The model under review builds one solid part; all positions refer to its coordinate system, in mm. A direction names the side the tool comes from. Coordinates: 2 decimals unless noted, no trailing zeros. Loops run counter-clockwise (first coordinate to the right, second up) from the corner with the lowest first, then second, coordinate; pieces in that order, holes last. Notation, with made-up numbers: (-25.75, 35.5) - (6.25, 35.5) arc R22 ccw to (6.25, 55.5) - close; hole circle Ø7 at (49.5, 52). An arc over 180 degrees is marked (long way). Use a Markdown table: item, result. Add a question column.
1) Add section B-B, the plane x = 205. Give the boundary of the cut face in (y, z), and give its area (3 significant figures).
2) Add section A-A, the plane z = -68. Give the boundary of the cut face in (x, y), and give its area (3 significant figures).
3) Add section C-C, the plane y = 62. Give the boundary of the cut face in (x, z).
4) Add section D-D, the plane z = -10. Give the boundary of the cut face in (x, y), and give its area (3 significant figures).
5) Clearance check with flat-ended pins moving along their axes: pin 1 (4 mm diameter, centred on x = 19.18, y = 96.25, fed in from -Z); pin 2 (1 mm diameter, centred on y = 67, z = 6, fed in from +X); pin 3 (4 mm diameter, centred on y = 31, z = -44.5, fed in from -X); pin 4 (10 mm diameter, centred on x = -85, z = -68, fed in from +Y). State where each tip first meets the part, or that it passes through.
6) To check wall thickness, follow L1, parallel to X at y = 39, z = -16; L2, parallel to Z at x = -150, y = 16; L3, parallel to Z at x = -205, y = 5. State the ranges of each line that lie inside material, in increasing order. Write a range as [from, to].
7) For faces 1 (the flat face through (-3, 62, -55)), 2 (the flat face through (-200, 62, 0)), 3 (the flat face through (-3, 62, 55)), 4 (the cylindrical face through (43, 89, 48)), list the 3-axis set-ups (+Z, -Z, +X, -X, +Y, -Y) from which the entire face can be reached by the end or side of a thin tool; tool diameter is ignored.
```python
from build123d import *

# Parameters (mm, degrees)
SKETCH1_W           = 450
SKETCH1_H           = 160
BOSS_EXTRUDE1_DEPTH = 10
SKETCH2_W           = 430
SKETCH2_H           = 110
SKETCH2_W_2         = 400
SKETCH2_H_2         = 80
BOSS_EXTRUDE2_DEPTH = 100
SKETCH3_R           = 5.5
CUT_EXTRUDE1_DEPTH  = 100
SKETCH4_R           = 21
CUT_EXTRUDE2_DEPTH  = 136
CIRPATTERN1_COUNT   = 6
CIRPATTERN2_COUNT   = 6
CIRPATTERN3_COUNT   = 6
FILLET1_R           = 5
SKETCH13_R          = 8
CUT_EXTRUDE3_DEPTH  = 100


with BuildPart() as part:
    # Sketch1 → Boss-Extrude1 (new body)
    with BuildSketch(Plane(origin=(0, 0, 0), x_dir=(1, 0, 0), z_dir=(0, 1, 0))):
        Rectangle(SKETCH1_W, SKETCH1_H)
    extrude(amount=BOSS_EXTRUDE1_DEPTH)

    # Sketch2 → Boss-Extrude2 (add)
    with BuildSketch(Plane(origin=(0, 10, 0), x_dir=(1, 0, 0), z_dir=(0, 1, 0))):
        Rectangle(SKETCH2_W, SKETCH2_H)
        Rectangle(SKETCH2_W_2, SKETCH2_H_2, mode=Mode.SUBTRACT)
    extrude(amount=BOSS_EXTRUDE2_DEPTH)

    # Sketch3 → Cut-Extrude1 (cut)
    with BuildSketch(Plane(origin=(0, 10, 0), x_dir=(1, 0, 0), z_dir=(0, 1, 0))):
        with Locations((-205, 68)):
            Circle(SKETCH3_R)
        with Locations((-85, 68)):
            Circle(SKETCH3_R)
        with Locations((-205, -68)):
            Circle(SKETCH3_R)
        with Locations((-85, -68)):
            Circle(SKETCH3_R)
        with Locations((205, 68)):
            Circle(SKETCH3_R)
        with Locations((85, 68)):
            Circle(SKETCH3_R)
        with Locations((85, -68)):
            Circle(SKETCH3_R)
        with Locations((205, -68)):
            Circle(SKETCH3_R)
    extrude(amount=-CUT_EXTRUDE1_DEPTH, mode=Mode.SUBTRACT)

    # Sketch4 → Cut-Extrude2 (cut, through all)
    with BuildSketch(Plane.XY.offset(55)):
        with Locations((-85, 110)):
            Circle(SKETCH4_R)
        with Locations((43, 110)):
            Circle(SKETCH4_R)
        with Locations((135, 110)):
            Circle(SKETCH4_R)
    extrude(amount=-CUT_EXTRUDE2_DEPTH, mode=Mode.SUBTRACT)

    # Sketch10 → M5 Tapped Hole1 (revolve, cut)
    with BuildSketch(Plane(origin=(158.815698604, 96.25, 55), x_dir=(0, -1, 0), z_dir=(1, 0, 0))):
        Polygon((0, 0), (0, 13.6618073), (2.1, 12.4), (2.1, 0.425), (2.525, 0), align=None)
    m5_tapped_hole1 = revolve(axis=Axis((158.815698604, 96.25, 61.35), (0, 0, -1)), mode=Mode.SUBTRACT)

    # Sketch11 → M5 Tapped Hole2 (revolve, cut)
    with BuildSketch(Plane(origin=(66.815698604, 96.25, 55), x_dir=(0, -1, 0), z_dir=(1, 0, 0))):
        Polygon((0, 0), (0, 13.6618073), (2.1, 12.4), (2.1, 0.425), (2.525, 0), align=None)
    m5_tapped_hole2 = revolve(axis=Axis((66.815698604, 96.25, 61.35), (0, 0, -1)), mode=Mode.SUBTRACT)

    # Sketch12 → M5 Tapped Hole3 (revolve, cut)
    with BuildSketch(Plane(origin=(-61.184301396, 96.25, 55), x_dir=(0, -1, 0), z_dir=(1, 0, 0))):
        Polygon((0, 0), (0, 13.6618073), (2.1, 12.4), (2.1, 0.425), (2.525, 0), align=None)
    m5_tapped_hole3 = revolve(axis=Axis((-61.184301396, 96.25, 61.35), (0, 0, -1)), mode=Mode.SUBTRACT)

    # CirPattern1: M5 Tapped Hole1 ×6 about axis, 3 skipped
    cirpattern1_axis = Axis((135, 110, -80), (0, 0, 1))
    add([m5_tapped_hole1.rotate(cirpattern1_axis, i * 360 / CIRPATTERN1_COUNT) for i in range(1, CIRPATTERN1_COUNT) if i not in (1, 2, 3)], mode=Mode.SUBTRACT)

    # CirPattern2: M5 Tapped Hole2 ×6 about axis, 3 skipped
    cirpattern2_axis = Axis((43, 110, -80), (0, 0, 1))
    add([m5_tapped_hole2.rotate(cirpattern2_axis, i * 360 / CIRPATTERN2_COUNT) for i in range(1, CIRPATTERN2_COUNT) if i not in (1, 2, 3)], mode=Mode.SUBTRACT)

    # CirPattern3: M5 Tapped Hole3 ×6 about axis, 3 skipped
    cirpattern3_axis = Axis((-85, 110, -80), (0, 0, 1))
    add([m5_tapped_hole3.rotate(cirpattern3_axis, i * 360 / CIRPATTERN3_COUNT) for i in range(1, CIRPATTERN3_COUNT) if i not in (1, 2, 3)], mode=Mode.SUBTRACT)

    # Mirror3: M5 Tapped Hole1, M5 Tapped Hole2, M5 Tapped Hole3 across plane
    add(m5_tapped_hole1.mirror(Plane.XY), mode=Mode.SUBTRACT)
    add(m5_tapped_hole2.mirror(Plane.XY), mode=Mode.SUBTRACT)
    add(m5_tapped_hole3.mirror(Plane.XY), mode=Mode.SUBTRACT)

    # Mirror3 copy 1 sketch → Mirror3 copy 1 (revolve, cut)
    with BuildSketch(Plane(origin=(111.184301396, 96.25, -55), x_dir=(-0.866025404, 0.5, 0), z_dir=(-0.5, -0.866025404, 0))):
        Polygon((0, 0), (0, -13.6618073), (2.1, -12.4), (2.1, -0.425), (2.525, 0), align=None)
    revolve(axis=Axis((111.184301396, 96.25, -61.35), (0, 0, -1)), mode=Mode.SUBTRACT)

    # Mirror3 copy 2 sketch → Mirror3 copy 2 (revolve, cut)
    with BuildSketch(Plane(origin=(135, 82.5, -55), x_dir=(-0.866025404, -0.5, 0), z_dir=(0.5, -0.866025404, 0))):
        Polygon((0, 0), (0, -13.6618073), (2.1, -12.4), (2.1, -0.425), (2.525, 0), align=None)
    revolve(axis=Axis((135, 82.5, -61.35), (0, 0, -1)), mode=Mode.SUBTRACT)

    # Mirror3 copy 3 sketch → Mirror3 copy 3 (revolve, cut)
    with BuildSketch(Plane(origin=(19.184301396, 96.25, -55), x_dir=(-0.866025404, 0.5, 0), z_dir=(-0.5, -0.866025404, 0))):
        Polygon((0, 0), (0, -13.6618073), (2.1, -12.4), (2.1, -0.425), (2.525, 0), align=None)
    revolve(axis=Axis((19.184301396, 96.25, -61.35), (0, 0, -1)), mode=Mode.SUBTRACT)

    # Mirror3 copy 4 sketch → Mirror3 copy 4 (revolve, cut)
    with BuildSketch(Plane(origin=(43, 82.5, -55), x_dir=(-0.866025404, -0.5, 0), z_dir=(0.5, -0.866025404, 0))):
        Polygon((0, 0), (0, -13.6618073), (2.1, -12.4), (2.1, -0.425), (2.525, 0), align=None)
    revolve(axis=Axis((43, 82.5, -61.35), (0, 0, -1)), mode=Mode.SUBTRACT)

    # Mirror3 copy 5 sketch → Mirror3 copy 5 (revolve, cut)
    with BuildSketch(Plane(origin=(-108.815698604, 96.25, -55), x_dir=(-0.866025404, 0.5, 0), z_dir=(-0.5, -0.866025404, 0))):
        Polygon((0, 0), (0, -13.6618073), (2.1, -12.4), (2.1, -0.425), (2.525, 0), align=None)
    revolve(axis=Axis((-108.815698604, 96.25, -61.35), (0, 0, -1)), mode=Mode.SUBTRACT)

    # Mirror3 copy 6 sketch → Mirror3 copy 6 (revolve, cut)
    with BuildSketch(Plane(origin=(-85, 82.5, -55), x_dir=(-0.866025404, -0.5, 0), z_dir=(0.5, -0.866025404, 0))):
        Polygon((0, 0), (0, -13.6618073), (2.1, -12.4), (2.1, -0.425), (2.525, 0), align=None)
    revolve(axis=Axis((-85, 82.5, -61.35), (0, 0, -1)), mode=Mode.SUBTRACT)

    # Fillet1
    fillet1_edges = [part.edges().sort_by_distance(p)[0] for p in [
        (0, 10, 40),
        (200, 10, 0),
        (0, 10, -40),
        (-200, 10, 0),
        (215, 10, 0),
        (215, 60, 55),
        (0, 10, -55),
        (215, 60, -55),
        (-215, 10, 0),
        (-215, 60, -55),
        (0, 10, 55),
        (-215, 60, 55),
        (200, 60, -40),
        (-200, 60, -40),
        (-200, 60, 40),
        (200, 60, 40),
    ]]
    fillet(fillet1_edges, radius=FILLET1_R)

    # Sketch13 → Cut-Extrude3 (cut)
    with BuildSketch(Plane.ZY.offset(215)):
        with Locations((-30, 30)):
            Circle(SKETCH13_R)
    extrude(amount=-CUT_EXTRUDE3_DEPTH, mode=Mode.SUBTRACT)


solid = part.part
```
From the geometry:
| question | item | result |
|---|---|---|
| 1 | outline | (0, -80) - (10, -80) - (10, -73.5) - (0, -73.5) - close; (0, -62.5) - (10, -62.5) - (10, -60) arc R5 cw to (15, -55) - (110, -55) - (110, 55) - (15, 55) arc R5 cw to (10, 60) - (10, 62.5) - (0, 62.5) - close; (0, 73.5) - (10, 73.5) - (10, 80) - (0, 80) - close |
| 1 | area | 12,400 mm^2 |
| 2 | outline | (-225, 0) - (-210.5, 0) - (-210.5, 10) - (-225, 10) - close; (-199.5, 0) - (-90.5, 0) - (-90.5, 10) - (-199.5, 10) - close; (-79.5, 0) - (79.5, 0) - (79.5, 10) - (-79.5, 10) - close; (90.5, 0) - (199.5, 0) - (199.5, 10) - (90.5, 10) - close; (210.5, 0) - (225, 0) - (225, 10) - (210.5, 10) - close |
| 2 | area | 4,060 mm^2 |
| 3 | outline | (-215, -50) arc R5 ccw to (-210, -55) - (210, -55) arc R5 ccw to (215, -50) - (215, 50) arc R5 ccw to (210, 55) - (-210, 55) arc R5 ccw to (-215, 50) - close; hole (-200, -35) arc R5 ccw to (-195, -40) - (195, -40) arc R5 ccw to (200, -35) - (200, 35) arc R5 ccw to (195, 40) - (-195, 40) arc R5 ccw to (-200, 35) - close |
| 4 | outline | (-225, 0) - (225, 0) - (225, 10) - (220, 10) arc R5 cw to (215, 15) - (215, 110) - (200, 110) - (200, 15) arc R5 cw to (195, 10) - (-195, 10) arc R5 cw to (-200, 15) - (-200, 110) - (-215, 110) - (-215, 15) arc R5 cw to (-220, 10) - (-225, 10) - close |
| 4 | area | 7,520 mm^2 |
| 5 | pin 1 | stops at z = -42.54 |
| 5 | pin 2 | stops at x = 215 |
| 5 | pin 3 | stops at x = -215 |
| 5 | pin 4 | passes through |
| 6 | L1 | x = [-215, -200], [200, 215] |
| 6 | L2 | z = [-55, -40], [40, 55] |
| 6 | L3 | z = [-80, -73.5], [-62.5, 62.5], [73.5, 80] |
| 7 | face 1 | -Z, +X, -X, +Y |
| 7 | face 2 | +Y |
| 7 | face 3 | +Z, +X, -X, +Y |
| 7 | face 4 | +Z, -Z, +Y |
